The model under review builds one solid part; all positions refer to its coordinate system, in mm. Face numbers are marked on the shaded views. A direction names the side the tool comes from. Round coordinates to 2 decimals unless told otherwise and drop trailing zeros. Loops run counter-clockwise (first coordinate to the right, second up) from the corner with the lowest first, then second, coordinate; pieces in that order, holes last. Notation, with made-up numbers: (64.5, -7.75) -> (102.5, -7.75) arc R20 ccw to (102.5, 7.25) -> close; hole circle Ø6 at (-30, 16.25). An arc over 180 degrees is marked (long way). Return JSON: item names as keys, results as strings. Group by question number.
```python
from build123d import *

# Parameters (mm, degrees)
CROQUIS1_R              = 3.1
SALIENTE_EXTRUIR1_DEPTH = 15
CROQUIS2_W              = 12.5
CROQUIS2_H              = 2.8
CORTAR_EXTRUIR1_DEPTH   = 13


with BuildPart() as part:
    # Croquis1 → Saliente-Extruir1 (new body)
    with BuildSketch(Plane.XY):
        with BuildLine():
            Line((0, 5.2), (20, 5.2))
            Line((20, 5.2), (20, -5.2))
            Line((20, -5.2), (0, -5.2))
            ThreePointArc((0, -5.2), (-5.2, 0), (0, 5.2))
        make_face()
        Circle(CROQUIS1_R, mode=Mode.SUBTRACT)
    extrude(amount=SALIENTE_EXTRUIR1_DEPTH)

    # Croquis2 → Cortar-Extruir1 (cut)
    with BuildSketch(Plane.XY.offset(15)):
        with Locations((13.75, 0)):
            Rectangle(CROQUIS2_W, CROQUIS2_H)
    extrude(amount=-CORTAR_EXTRUIR1_DEPTH, mode=Mode.SUBTRACT)


solid = part.part
```
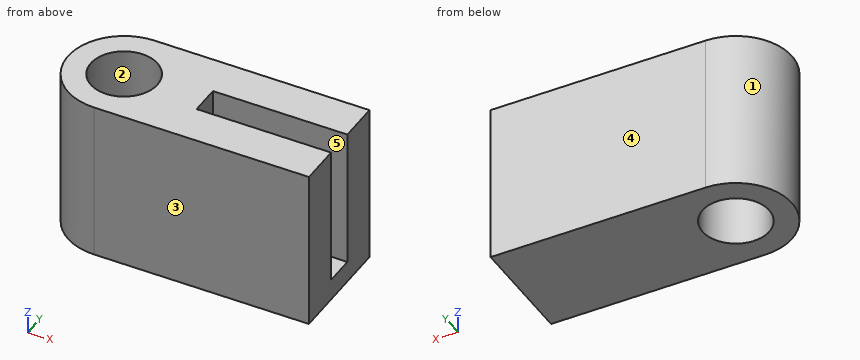
1. We need section A-A, the plane z = 8.75. Write out the cut boundary in (x, y), then the cut area to 3 significant figures.
2. Draft analysis for pull direction X (two halves, no side actions). For the marked faces 1, 2 and 3, state which applies: pulls with the +X half, pulls with the -X half, needs draft (parallel to the pull), parting line crosses it, or undercut.
3. For P1, Ø1.4, axis at y = -0.5, z = 5.5, coming from the +X side; P2, Ø5.5, axis at x = 0, y = 0, coming from the +Z side; P3, Ø1.4, axis at x = 11, y = 0, coming from the +Z side, all flat-tipped, find the tip position at first contact; note any pin that passes through.
4. We need section D-D, the plane y = 2.5. Write out the cut boundary in (x, z).
5. We need section C-C, the plane x = -2.5. Write out the cut boundary in (y, z).
6. We need section B-B, the plane y = 0. Write out the cut boundary in (x, z).
7. Wall thickness on line 1 (Y direction, x = 0, z = 4.5); line 2 (Y direction, x = 13, z = 5); line 3 (X direction, y = -1.5, z = 3): over which ranges is each line inside the solid? List them lowest first.
8. Tool access review of the marked faces 4 and 5: name each direction out of +Z, -Z, +X, -X, +Y, -Y from which nothing blocks a thin tool from reaching the whole face with its end or side.
Check sheet entries:
{
 "1": {"outline": "(0, -5.2) -> (20, -5.2) -> (20, -1.4) -> (7.5, -1.4) -> (7.5, 1.4) -> (20, 1.4) -> (20, 5.2) -> (0, 5.2) arc R5.2 ccw to start; hole circle Ø6.2 at (0, 0)", "area": "185 mm²"},
 "2": {"face 1": "pulls with the -X half", "face 2": "undercut", "face 3": "needs draft"},
 "3": {"P1": "stops at x = 7.5", "P2": "passes through", "P3": "stops at z = 2"},
 "4": {"outline": "(-4.56, 0) -> (-1.83, 0) -> (-1.83, 15) -> (-4.56, 15) -> close; (1.83, 0) -> (20, 0) -> (20, 15) -> (1.83, 15) -> close"},
 "5": {"outline": "(-4.56, 0) -> (-1.83, 0) -> (-1.83, 15) -> (-4.56, 15) -> close; (1.83, 0) -> (4.56, 0) -> (4.56, 15) -> (1.83, 15) -> close"},
 "6": {"outline": "(-5.2, 0) -> (-3.1, 0) -> (-3.1, 15) -> (-5.2, 15) -> close; (3.1, 0) -> (20, 0) -> (20, 2) -> (7.5, 2) -> (7.5, 15) -> (3.1, 15) -> close"},
 "7": {"line 1": "y = -5.2 to -3.1, 3.1 to 5.2", "line 2": "y = -5.2 to -1.4, 1.4 to 5.2", "line 3": "x = -4.98 to -2.71, 2.71 to 20"},
 "8": {"face 4": "+Z, -Z, +X, -X, +Y", "face 5": "+Z, +X"}
}
